Part print with two shaded views. Sizes in mm from the minimum x, y, z corner. A direction names the side the tool comes from. Round coordinates to 2 decimals unless told otherwise and drop trailing zeros. Loops run counter-clockwise (first coordinate to the right, second up) from the corner with the lowest first, then second, coordinate; pieces in that order, holes last. Notation, with made-up numbers: (-19.75, 29) -> (12.25, 29) arc R8 ccw to (12.25, 36) -> close; hole circle Ø8 at (8.5, 85.25). An arc over 180 degrees is marked (long way). Use a Markdown table: item, result. Add a question column.
Item 1: Which spindle directions (+Z, -Z, +X, -X, +Y, -Y) get a long thin tool onto all of the face, cutting with end or side? Do the marked faces 1 and 2. Say none if no direction does.
Item 2: Probe line 1 (X direction, y = 0.9, z = 15); line 2 (Y direction, x = 54, z = 42.9); line 3 (Z direction, x = 6, y = 2). List the from-to ranges inside material, lowest first. Write a range as [from, to].
Item 3: Cut at A-A, the plane z = 28.5. List the corners of the cut face in (x, y) (3 decimals).
Item 4: Flat gauge pins, fed straight in: pin 1 (6.5 mm diameter, centred on x = 55, z = 15, fed in from +Y) (3 decimals); pin 2 (12 mm diameter, centred on x = 54, y = 17.5, fed in from -Z). Where does each tip first touch, or does it go through?
Item 5: Cut at C-C, the plane y = 44. List the corners of the cut face in (x, z).
Item 6: Cut at B-B, the plane x = 38.5. List the corners of the cut face in (y, z) (3 decimals).
Item 7: Cut at D-D, the plane z = 15. List the corners of the cut face in (x, y) (3 decimals), plus the area to 3 significant figures.
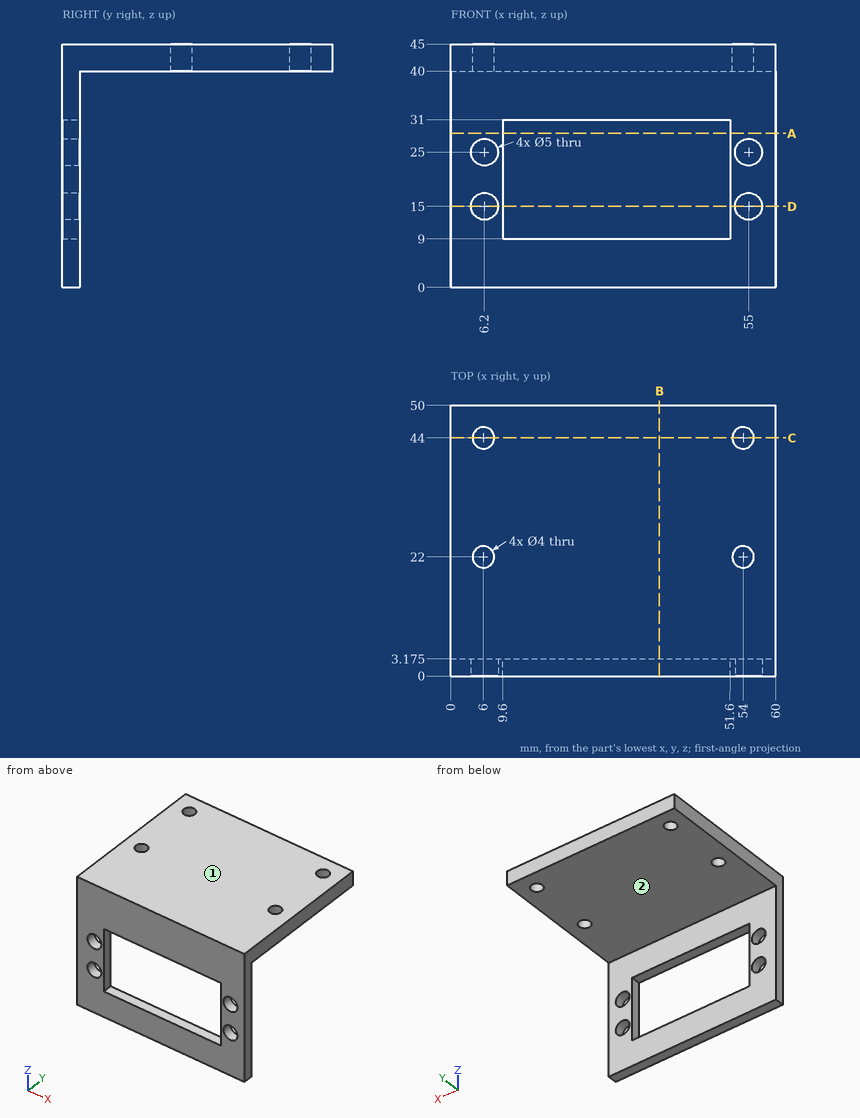
A:
| question | item | result |
|---|---|---|
| 1 | face 1 | +Z, +X, -X, +Y, -Y |
| 1 | face 2 | -Z, +X, -X, +Y |
| 2 | line 1 | x = [0, 3.7], [8.7, 9.6], [51.6, 52.5], [57.5, 60] |
| 2 | line 2 | y = [0, 20], [24, 42], [46, 50] |
| 2 | line 3 | z = [0, 12.51], [17.49, 22.51], [27.49, 45] |
| 3 | outline | (0, 0) -> (9.6, 0) -> (9.6, 3.175) -> (0, 3.175) -> close; (51.6, 0) -> (60, 0) -> (60, 3.175) -> (51.6, 3.175) -> close |
| 4 | pin 1 | stops at y = 3.175 |
| 4 | pin 2 | stops at z = 40 |
| 5 | outline | (0, 40) -> (4, 40) -> (4, 45) -> (0, 45) -> close; (8, 40) -> (52, 40) -> (52, 45) -> (8, 45) -> close; (56, 40) -> (60, 40) -> (60, 45) -> (56, 45) -> close |
| 6 | outline | (0, 0) -> (3.175, 0) -> (3.175, 9) -> (0, 9) -> close; (0, 31) -> (3.175, 31) -> (3.175, 40) -> (50, 40) -> (50, 45) -> (0, 45) -> close |
| 7 | outline | (0, 0) -> (3.7, 0) -> (3.7, 3.175) -> (0, 3.175) -> close; (8.7, 0) -> (9.6, 0) -> (9.6, 3.175) -> (8.7, 3.175) -> close; (51.6, 0) -> (52.5, 0) -> (52.5, 3.175) -> (51.6, 3.175) -> close; (57.5, 0) -> (60, 0) -> (60, 3.175) -> (57.5, 3.175) -> close |
| 7 | area | 25.4 mm^2 |
